Can you work these out from the model? Positions are in its coordinate system, mm. Face numbers are marked on the shaded views. A direction names the side the tool comes from. Coordinates: 2 decimals unless noted, no trailing zeros. Loops run counter-clockwise (first coordinate to the right, second up) from the corner with the lowest first, then second, coordinate; pieces in that order, holes last. Notation, with made-up numbers: M 77,57.25 L 113,57.25 A28 cw 113,77.25 Z; hole C 9.5,10 d6. An arc over 180 degrees is marked long. Return JSON: item names as keys, results as strings. Group by question number.
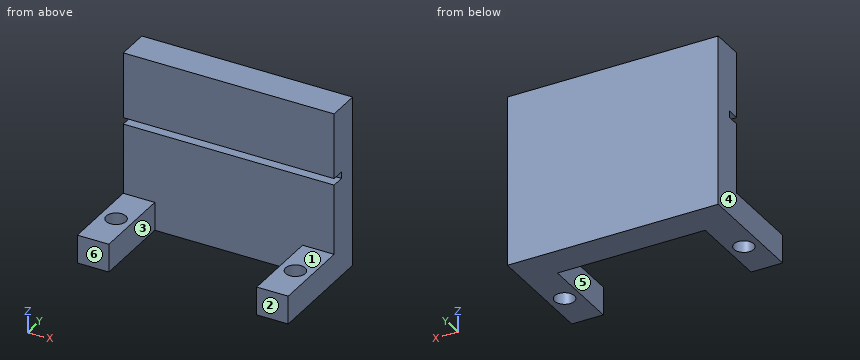
Autodesk Inventor part; units mm, degrees
ref_plane "YZ Plane" through (0, 0, 0) normal (1, 0, 0) x (0, 1, 0)
ref_plane "XZ Plane" through (0, 0, 0) normal (0, 1, 0) x (-1, 0, 0)
ref_plane "XY Plane" through (0, 0, 0) normal (0, 0, 1) x (1, 0, 0)
sketch "草圖1" plane through (0, 0, 0) normal (0, 0, 1) x (1, 0, 0)
  line L0 (0, 0) -> (32.1, 0)
  line L1 (32.1, 0) -> (32.1, 12.4)
  line L2 (32.1, 12.4) -> (0, 12.4)
  line L3 (0, 12.4) -> (0, 0)
  line L4 (4.8, 12.4) -> (4.8, 0)
  line L5 (27.3, 12.4) -> (27.3, 0)
  line L6 (32.1, 12.4) -> (0, 12.4)
  line L7 (0, 12.4) -> (0, 17.4)
  line L8 (0, 17.4) -> (32.1, 17.4)
  line L9 (32.1, 17.4) -> (32.1, 12.4)
  circle A0 centre (2.4, 6.2) radius 1.5
  circle A1 centre (29.7, 6.2) radius 1.5
  point P0 (0, 12.4)
  dimension "d0" = 12.4
  dimension "d1" = 32.1
  dimension "d2" = 4.8
  dimension "d3" = 4.8
  dimension "d6" = 5
  dimension "d7" = 32.1
  dimension "d14" = 6.2
  dimension "d15" = 6.2
  dimension "d16" = 2.4
  dimension "d17" = 2.4
  dimension "d18" = 3
  dimension "d19" = 3
extrude "擠出1" add sketch "草圖1" along normal blind 4.3 contours L3 L2 L4 L0 | L5 L2 L1 L0 | A0 | A1
extrude "擠出2" add sketch "草圖1" along normal blind 15 contours L7 L8 L9 L2
sketch "草圖2" plane through (0, 0, 15) normal (0, 0, 1) x (1, 0, 0)
  line L0 (32.1, 17.4) -> (0, 17.4)
  line L1 (0, 17.4) -> (0, 12.4)
  line L2 (0, 12.4) -> (32.1, 12.4)
  line L3 (32.1, 12.4) -> (32.1, 17.4)
  line L4 (0, 17.4) -> (32.1, 17.4)
  line L5 (32.1, 17.4) -> (32.1, 14.9)
  line L6 (0, 11.4) -> (0, 17.4)
  line L7 (0, 14.4) -> (32.1, 14.4)
  point P0 (0, 0)
  dimension "d22" = 2
extrude "擠出3" add sketch "草圖2" along normal blind 1 contours L3 L7 L1 L0
sketch "草圖3" plane through (0, 0, 16) normal (0, 0, 1) x (1, 0, 0)
  line L0 (32.1, 14.4) -> (32.1, 17.4)
  line L1 (32.1, 17.4) -> (0, 17.4)
  line L2 (0, 17.4) -> (0, 14.4)
  line L3 (0, 14.4) -> (0, 12.4)
  line L4 (0, 12.4) -> (32.1, 12.4)
  line L5 (32.1, 12.4) -> (32.1, 14.4)
  line L6 (0, 12.4) -> (32.1, 12.4)
  line L7 (32.1, 12.4) -> (32.1, 17.4)
  line L8 (32.1, 17.4) -> (0, 17.4)
  line L9 (0, 17.4) -> (0, 12.4)
  line L10 (32.1, 14.4) -> (0, 14.4)
  line L11 (0, 14.4) -> (32.1, 14.4)
  point P0 (0, 0)
extrude "擠出4" add sketch "草圖3" along normal blind 10
extrude "擠出5" cut sketch "草圖1" along normal through all contours A0 | A1
properties part number "固定塊"
1) Suppose I cut it at C-C, the plane y = 6.2. List the corners of the cut face in (x, z) for me, then the cut area to 3 significant figures.
2) For the marked faces 1, 2 and 3, which set-ups out of +Z, -Z, +X, -X, +Y, -Y let a thin tool reach every point of the face, with its end or its side?
3) For pin 1 (11 mm diameter, centred on x = 9.5, z = 20, fed in from -Y); pin 2 (2 mm diameter, centred on y = 6.5, z = 1.5, fed in from -X); pin 3 (1.4 mm diameter, centred on x = 28.5, y = 3, fed in from +Z); pin 4 (1.8 mm diameter, centred on x = 29.7, y = 6.2, fed in from +Z), each with a flat end and sliding along its axis, tell me the tip position at first contact or that it passes through.
4) If we mould it in two halves opening along X, with no side actions, what happens to the marked faces 4, 5 and 6? For each: +X half, -X half, draft (parallel to the pull), parting line (faces both ways), or undercut.
5) If I drill on line 1 (X direction, y = 6.2, z = 3.2); line 2 (Y direction, x = 29.7, z = 1.15); line 3 (Z direction, x = 20, y = 13.5), over which ranges is the centre line in solid material (lowest first)? Write a range as from..to.
6) Suppose I cut it at B-B, the plane x = 29.7. List the corners of the cut face in (y, z) for me.
7) Suppose I cut it at A-A, the plane y = 3.25. List the corners of the cut face in (x, z) for me, then the cut area to 3 significant figures.
8) Suppose I cut it at D-D, the plane z = 2. List the corners of the cut face in (x, y) for me, then the cut area to 3 significant figures.
Returned:
{
 "1": {"outline": "M 0,0 L 0.9,0 L 0.9,4.3 L 0,4.3 Z; M 3.9,0 L 4.8,0 L 4.8,4.3 L 3.9,4.3 Z; M 27.3,0 L 28.2,0 L 28.2,4.3 L 27.3,4.3 Z; M 31.2,0 L 32.1,0 L 32.1,4.3 L 31.2,4.3 Z", "area": "15.5 mm²"},
 "2": {"face 1": "+Z, +X, -X, -Y", "face 2": "+Z, -Z, +X, -X, -Y", "face 3": "+Z, -Z, -Y"},
 "3": {"pin 1": "stops at y = 12.4", "pin 2": "stops at x = 0", "pin 3": "stops at z = 4.3", "pin 4": "passes through"},
 "4": {"face 4": "-X half", "face 5": "undercut", "face 6": "draft"},
 "5": {"line 1": "x = 0..0.9, 3.9..4.8, 27.3..28.2, 31.2..32.1", "line 2": "y = 0..4.7, 7.7..17.4", "line 3": "z = 0..15, 16..26"},
 "6": {"outline": "M 0,0 L 4.7,0 L 4.7,4.3 L 0,4.3 Z; M 7.7,0 L 17.4,0 L 17.4,26 L 12.4,26 L 12.4,16 L 14.4,16 L 14.4,15 L 12.4,15 L 12.4,4.3 L 7.7,4.3 Z"},
 "7": {"outline": "M 0,0 L 4.8,0 L 4.8,4.3 L 0,4.3 Z; M 27.3,0 L 32.1,0 L 32.1,4.3 L 27.3,4.3 Z", "area": "41.3 mm²"},
 "8": {"outline": "M 0,0 L 4.8,0 L 4.8,12.4 L 27.3,12.4 L 27.3,0 L 32.1,0 L 32.1,17.4 L 0,17.4 Z; hole C 2.4,6.2 d3; hole C 29.7,6.2 d3", "area": "265 mm²"}
}
